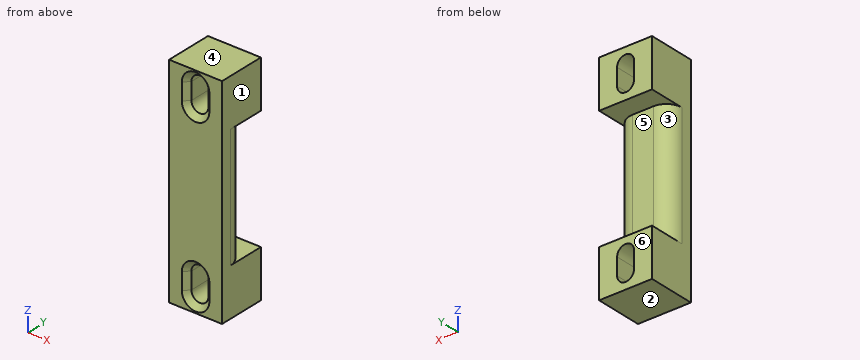
from build123d import *

# Parameters (mm, degrees)
F0_W     = 10
F0_H     = 41
F1_DEPTH = 5
F4_DEPTH = 23
F6_DEPTH = 4
F7_SIZE  = 1


with BuildPart() as f1:
    # F0 (on Front) → F1 (new body)
    with BuildSketch(Plane.XZ):
        with Locations((5, 20.5)):
            Rectangle(F0_W, F0_H)
        with BuildLine():
            ThreePointArc((3.4, 6.1), (5, 7.7), (6.6, 6.1))
            Line((6.6, 6.1), (6.6, 2.9))
            ThreePointArc((6.6, 2.9), (5, 1.3), (3.4, 2.9))
            Line((3.4, 2.9), (3.4, 6.1))
        make_face(mode=Mode.SUBTRACT)
        with BuildLine():
            ThreePointArc((6.6, 34.9), (5, 33.3), (3.4, 34.9))
            Line((3.4, 34.9), (3.4, 38.1))
            ThreePointArc((3.4, 38.1), (5, 39.7), (6.6, 38.1))
            Line((6.6, 38.1), (6.6, 34.9))
        make_face(mode=Mode.SUBTRACT)
    extrude(amount=F1_DEPTH)

    # F3 (on offset) → F4 (cut)
    with BuildSketch(Plane.XY.offset(9)):
        with BuildLine():
            Line((10, 0), (7, 0))
            ThreePointArc((7, 0), (9.12132, -0.87868), (10, -3))
            Line((10, -3), (10, -2.5))
            Line((10, -2.5), (10, 0))
        make_face()
        with BuildLine():
            ThreePointArc((0, -3), (0.87868, -0.87868), (3, 0))
            Line((3, 0), (0, 0))
            Line((0, 0), (0, -3))
        make_face()
    extrude(amount=F4_DEPTH, mode=Mode.SUBTRACT)

    # F5 (on face) → F6 (join)
    with BuildSketch(Plane(origin=(0, 0, 0), x_dir=(-1, 0, 0), z_dir=(0, 1, 0))):
        Polygon((0, 32), (0, 41), (-10, 41), (-10, 32), (-7, 32), (-3, 32), align=None)
        with BuildLine():
            Line((-6.6, 34.9), (-6.6, 38.1))
            ThreePointArc((-6.6, 38.1), (-5, 39.7), (-3.4, 38.1))
            Line((-3.4, 38.1), (-3.4, 34.9))
            ThreePointArc((-3.4, 34.9), (-5, 33.3), (-6.6, 34.9))
        make_face(mode=Mode.SUBTRACT)
        Polygon((0, 9), (-3, 9), (-7, 9), (-10, 9), (-10, 0), (0, 0), align=None)
        with BuildLine():
            Line((-6.6, 2.9), (-6.6, 6.1))
            ThreePointArc((-6.6, 6.1), (-5, 7.7), (-3.4, 6.1))
            Line((-3.4, 6.1), (-3.4, 2.9))
            ThreePointArc((-3.4, 2.9), (-5, 1.3), (-6.6, 2.9))
        make_face(mode=Mode.SUBTRACT)
    extrude(amount=F6_DEPTH)

    # F7
    f7_edges = [f1.edges().sort_by_distance(p)[0] for p in [
        (5, -5, 33.3),
        (5, -5, 1.3),
    ]]
    chamfer(f7_edges, length=F7_SIZE)


solid = f1.part
Could you check a few things on this model? Use its own coordinates, in mm. Face numbers are marked on the shaded views. A direction names the side the tool comes from. Give positions to 0.01 mm unless a question says otherwise; leave off trailing zeros. Order: outer loops, then holes, each group sorted by start corner. A loop starts at its lowest first (then second) coordinate and runs counter-clockwise, first axis right, second up. Notation, with made-up numbers: (36, -13.75) -> (90, -13.75) arc R8 cw to (90, -8.75) -> close; hole circle Ø3 at (27.5, -6). An arc over 180 degrees is marked (long way). Return JSON: item names as keys, results as strings.
1. Thinking about a two-plate mould opening in Z: for the marked faces 1, 2, 3 and 4, which applies, pulls with the +Z half, pulls with the -Z half, needs draft (parallel to the pull), parting line crosses it, or undercut?
Answer list:
{"face 1": "needs draft", "face 2": "pulls with the -Z half", "face 3": "undercut", "face 4": "pulls with the +Z half"}
2. Imagine slicing it at A-A on y = 0.75. List the corners of the cut face in (x, z) for me.
Answer list:
{"outline": "(0, 0) -> (10, 0) -> (10, 9) -> (0, 9) -> close; (0, 32) -> (10, 32) -> (10, 41) -> (0, 41) -> close; hole (3.4, 2.9) arc R1.6 ccw to (6.6, 2.9) -> (6.6, 6.1) arc R1.6 ccw to (3.4, 6.1) -> close; hole (3.4, 34.9) arc R1.6 ccw to (6.6, 34.9) -> (6.6, 38.1) arc R1.6 ccw to (3.4, 38.1) -> close"}
3. For pin 1 Ø3 at (x, z) = (6, 20) entering from +Y; pin 2 Ø4 at (y, z) = (-0.5, 29) entering from -X, each with a flat end and sliding along its axis, tell me the tip position at first contact or that it passes through.
Answer list:
{"pin 1": "stops at y = 0", "pin 2": "stops at x = 0.04"}
4. Imagine slicing it at B-B on x = 5. List the corners of the cut face in (y, z) for me.
Answer list:
{"outline": "(-5, 0) -> (4, 0) -> (4, 1.3) -> (-4, 1.3) -> (-5, 0.3) -> close; (-5, 8.7) -> (-4, 7.7) -> (4, 7.7) -> (4, 9) -> (0, 9) -> (0, 32) -> (4, 32) -> (4, 33.3) -> (-4, 33.3) -> (-5, 32.3) -> close; (-5, 40.7) -> (-4, 39.7) -> (4, 39.7) -> (4, 41) -> (-5, 41) -> close"}
5. Imagine slicing it at D-D on z = 30. List the corners of the cut face in (x, y) for me, then the cut area to 3 significant figures.
Answer list:
{"outline": "(0, -5) -> (10, -5) -> (10, -3) arc R3 ccw to (7, 0) -> (3, 0) arc R3 ccw to (0, -3) -> close", "area": "46.1 mm2"}
6. On a 3-axis mill with a long thin cutter (end or side, diameter ignored), from which of +Z, -Z, +X, -X, +Y, -Y can I reach the whole of each face in a straight line? I mean the marked faces 5 and 6. Say none if no direction works.
Answer list:
{"face 5": "+X, -X, +Y", "face 6": "+Z, -Z, +X, -X, +Y"}
7. I need wall thicknesses on line 1 (Z direction, x = 7.25, y = 1.5); line 2 (X direction, y = 1.25, z = 35); line 3 (Z direction, x = 3.75, y = -0.5). Which ranges of each line are inside material? Lowest first, please. Write a range as from..to.
Answer list:
{"line 1": "z = 0..9, 32..41", "line 2": "x = 0..3.4, 6.6..10", "line 3": "z = 0..1.9, 7.1..33.9, 39.1..41"}
8. Imagine slicing it at C-C on y = -3.5. List the corners of the cut face in (x, z) for me, then the cut area to 3 significant figures.
Answer list:
{"outline": "(0, 0) -> (10, 0) -> (10, 41) -> (0, 41) -> close; hole (3.4, 2.9) arc R1.6 ccw to (6.6, 2.9) -> (6.6, 6.1) arc R1.6 ccw to (3.4, 6.1) -> close; hole (3.4, 34.9) arc R1.6 ccw to (6.6, 34.9) -> (6.6, 38.1) arc R1.6 ccw to (3.4, 38.1) -> close", "area": "373 mm2"}
